from build123d import *

# Parameters (mm, degrees)
MAIN_BODY_DEPTH                        = 7
FLANG_CUT_RIGHT_DEPTH                  = 2.754419
FLANG_CUT_RIGHT_DIRECTION_2_REACH      = 15.268
FLANG_CUT_RIGHT_DIRECTION_2_END_RADIUS = 6
FLANG_CUT_LEFT_DEPTH                   = 2.754419
FLANG_CUT_LEFT_DIRECTION_2_REACH       = 17.116
FLANG_CUT_LEFT_DIRECTION_2_END_RADIUS  = 6
GUIDE_CUTS_DEPTH                       = 14.586908947


# Read off the part's stored shape, not the designer's step: CSK SLOT for M1.6 Countersunk Flat Head Screw9
with BuildPart() as part:
    # Sketch1 → main body (new body)
    with BuildSketch(Plane(origin=(0, 0, 0), x_dir=(1, 0, 0), z_dir=(0, 1, 0))):
        with BuildLine():
            Line((-0.042515674, 6.696868743), (-2.796934729, 6.696868743))
            ThreePointArc((-2.796934729, 6.696868743), (-1.044786012, 2.204228056), (3.447854676, 0.452079339))
            Line((3.447854676, 0.452079339), (3.447854676, 3.206498394))
            ThreePointArc((3.447854676, 3.206498394), (0.899757637, 4.148771704), (-0.042515674, 6.696868743))
        make_face()
        with BuildLine():
            Line((1.415300329, 6.696868743), (-0.042515674, 6.696868743))
            ThreePointArc((-0.042515674, 6.696868743), (0.899757637, 4.148771704), (3.447854676, 3.206498394))
            Line((3.447854676, 3.206498394), (3.447854676, 4.664314396))
            ThreePointArc((3.447854676, 4.664314396), (1.925062469, 5.174076537), (1.415300329, 6.696868743))
        make_face()
        with BuildLine():
            ThreePointArc((6.447854676, 6.446868743), (3.322947371, 9.694460438), (-0.042515674, 6.696868743))
            Line((-0.042515674, 6.696868743), (1.415300329, 6.696868743))
            ThreePointArc((1.415300329, 6.696868743), (1.907300469, 7.701647544), (2.897854676, 8.221692678))
            ThreePointArc((2.897854676, 8.221692678), (4.470646882, 7.719660949), (4.972678611, 6.146868743))
            ThreePointArc((4.972678611, 6.146868743), (4.452633477, 5.156314537), (3.447854676, 4.664314396))
            Line((3.447854676, 4.664314396), (3.447854676, 3.206498394))
            ThreePointArc((3.447854676, 3.206498394), (5.582702679, 4.238928527), (6.447854676, 6.446868743))
        make_face()
    extrude(amount=MAIN_BODY_DEPTH)

    # Sketch15 → flang cut right (cut)
    with BuildSketch(Plane(origin=(0, 0, -0.452079339), x_dir=(0, -1, 0), z_dir=(0, 0, 1))):
        Polygon((0, 3.447854676), (0, 2.712125029), (-7, 3.447854676), align=None)
    extrude(amount=-FLANG_CUT_RIGHT_DEPTH, mode=Mode.SUBTRACT)

    # flang cut right direction 2: up to this cylinder (the profile starts inside it)
    flang_cut_right_direction_2_end = Plane(origin=(3.197854676, 2.333333, -6.446868743), z_dir=(0, -1, 0)) * Cylinder(FLANG_CUT_RIGHT_DIRECTION_2_END_RADIUS, 43.536, mode=Mode.PRIVATE)
    # Sketch15 → flang cut right direction 2 (cut, up to the surface)
    with BuildSketch(Plane(origin=(0, 0, -0.452079339), x_dir=(0, -1, 0), z_dir=(0, 0, 1)), mode=Mode.PRIVATE) as flang_cut_right_direction_2_sk1:
        Polygon((0, 3.447854676), (0, 2.712125029), (-7, 3.447854676), align=None)
    flang_cut_right_direction_2_tool1 = extrude(flang_cut_right_direction_2_sk1.sketch, amount=FLANG_CUT_RIGHT_DIRECTION_2_REACH, mode=Mode.PRIVATE) & flang_cut_right_direction_2_end
    add(flang_cut_right_direction_2_tool1.solids().sort_by_distance((3.202611, 2.333333, -0.452079))[0], mode=Mode.SUBTRACT)

    # Sketch13 → flang cut left (cut)
    with BuildSketch(Plane(origin=(-2.796934729, 0, 0), x_dir=(0, 0, -1), z_dir=(1, 0, 0))):
        Polygon((6.696868743, 0), (6.696868743, 7), (5.7130829, 0), align=None)
    extrude(amount=FLANG_CUT_LEFT_DEPTH, mode=Mode.SUBTRACT)

    # flang cut left direction 2: up to this cylinder (the profile starts inside it)
    flang_cut_left_direction_2_end = Plane(origin=(3.197854676, 2.333333, -6.446868743), z_dir=(0, -1, 0)) * Cylinder(FLANG_CUT_LEFT_DIRECTION_2_END_RADIUS, 47.232, mode=Mode.PRIVATE)
    # Sketch13 → flang cut left direction 2 (cut, up to the surface)
    with BuildSketch(Plane(origin=(-2.796934729, 0, 0), x_dir=(0, 0, -1), z_dir=(1, 0, 0)), mode=Mode.PRIVATE) as flang_cut_left_direction_2_sk1:
        Polygon((6.696868743, 0), (6.696868743, 7), (5.7130829, 0), align=None)
    flang_cut_left_direction_2_tool1 = extrude(flang_cut_left_direction_2_sk1.sketch, amount=-FLANG_CUT_LEFT_DIRECTION_2_REACH, mode=Mode.PRIVATE) & flang_cut_left_direction_2_end
    add(flang_cut_left_direction_2_tool1.solids().sort_by_distance((-2.796935, 2.333333, -6.36894))[0], mode=Mode.SUBTRACT)

    # CSK SLOT for M1.6 Countersunk Flat H 2 → CSK SLOT for M1.6 Countersunk Flat Head Screw9 (revolve, cut)
    with BuildSketch(Plane(origin=(-1.673520994, 3.5, -1.59907768), x_dir=(0.723004631868789, 0, 0.6908431821305592), z_dir=(0, 1, 0))):
        Polygon((0.9, 4.170332063), (0.9, 5.425223714), (0, 5.425223714), (0, 0.870183673), (1.8, 0.870183673), (1.8, 3.270332063), align=None)
    revolve(axis=Axis((-1.673520994, 3.5, -1.59907768), (0.6908431821305593, 0, -0.7230046318687892)), mode=Mode.SUBTRACT)

    # Sketch11 → guide cuts (cut, through all)
    with BuildSketch(Plane.XZ):
        with BuildLine():
            Line((1.060664016, -5.013453966), (1.614472941, -5.59077162))
            ThreePointArc((1.614472941, -5.59077162), (1.951784592, -5.147904022), (2.408284716, -4.829284347))
            Line((2.408284716, -4.829284347), (1.85447579, -4.251966693))
            Line((1.85447579, -4.251966693), (1.060664016, -5.013453966))
        make_face()
        with BuildLine():
            Line((5.335045336, -7.88028352), (4.78123641, -7.302965866))
            ThreePointArc((4.78123641, -7.302965866), (4.443924759, -7.745833465), (3.987424635, -8.064453139))
            Line((3.987424635, -8.064453139), (4.541233561, -8.641770793))
            Line((4.541233561, -8.641770793), (5.335045336, -7.88028352))
        make_face()
    extrude(amount=-GUIDE_CUTS_DEPTH, mode=Mode.SUBTRACT)


solid = part.part
Could you check a few things on this model? Use its own coordinates, in mm. A direction names the side the tool comes from. Give positions to 0.01 mm unless a question says otherwise; leave off trailing zeros. Order: outer loops, then holes, each group sorted by start corner. A loop starts at its lowest first (then second) coordinate and runs counter-clockwise, first axis right, second up. Notation, with made-up numbers: (28, 43.5) - (35, 43.5) arc R13 ccw to (35, 49.5) - close; hole circle Ø10 at (48, -14). An arc over 180 degrees is marked (long way). One line per question, with ' | ' between items. Start each with the question number.
Item 1: I need wall thicknesses on probe 1 along Z at (x, y) = (4.5, 4.5); probe 2 along X at (y, z) = (2.5, -6.25); probe 3 along X at (y, z) = (2.75, -7). Which ranges of each line are inside material? Lowest first, please. Write a range as [from, to].
Item 2: Thinking about a two-plate mould opening in Y: for faces 3 (the flat face through (-1.4, 3.55, -6.21)), 4 (the cylindrical face through (1.01, 2.96, -1.92)), 5 (the flat face through (2, 7, -4)), 6 (the flat face through (-0.043, 2, -6.4)), which applies, pulls with the +Y half, pulls with the -Y half, needs draft (parallel to the pull), parting line crosses it, or undercut?
Item 3: I want a section at A-A on z = -7.75. Write out the boundary of the cut face in (x, y), then the cut area to 3 significant figures.
Item 4: I'm going to push flat-ended pins straight in: pin 1 Ø0.8 at (y, z) = (5, -6) entering from -X; pin 2 Ø1.5 at (y, z) = (1, -8) entering from +X; pin 3 Ø1.5 at (x, y) = (-1.5, 2) entering from +Z; pin 4 Ø2 at (x, y) = (5.5, 1.5) entering from -Z. Where does each tip first touch, or does it pass through?
Item 5: I want a section at D-D on y = 5.75. Write out the boundary of the cut face in (x, z), then the cut area to 3 significant figures.
Item 6: I want a section at B-B on x = 4.25. Write out the boundary of the cut face in (y, z), then the cut area to 3 significant figures.
Item 7: I want a section at C-C on y = 0.75. Write out the boundary of the cut face in (x, z).
Item 8: For faces 1 (the flat face through (0.8, 0, -5.1)), 2 (the flat face through (3.075, 3.451, -1.807)), which set-ups out of +Z, -Z, +X, -X, +Y, -Y let a thin tool reach every point of the face, with its end or its side?
Verdict:
1) probe 1: [-9.42, -8.6], [-5.2, -3.47] | probe 2: [-0.04, 1.41], [4.99, 6.44] | probe 3: [0, 1.48], [4.91, 6.4]
2) face 3: pulls with the -Y half | face 4: undercut | face 5: pulls with the +Y half | face 6: needs draft
3) outline: (0.22, 0) - (1.96, 0) - (1.96, 7) - (0.22, 7) - close; (5.21, 0) - (6.18, 0) - (6.18, 7) - (5.21, 7) - close | area: 18.9 mm^2
4) pin 1: x = -2.8 | pin 2: x = 6.35 | pin 3: z = -1.97 | pin 4: z = -9.42
5) outline: (-2.8, -6.52) - (-0.04, -6.52) - (-0.04, -6.7) arc R3.25 ccw (long way) to (3.45, -3.21) - (3.32, -3.21) - (3.32, -0.45) arc R6 ccw to start; hole (1.06, -5.01) - (1.61, -5.59) arc R1.8 ccw to (3.99, -8.06) - (4.54, -8.64) - (5.34, -7.88) - (4.78, -7.3) arc R1.8 ccw to (2.41, -4.83) - (1.85, -4.25) - close | area: 41.9 mm^2
6) outline: (0, -9.52) - (7, -9.52) - (7, -8.34) - (0, -8.34) - close; (0, -4.99) - (7, -4.99) - (7, -3.37) - (0, -3.37) - close | area: 19.6 mm^2
7) outline: (-2.77, -5.82) - (-0.04, -5.82) - (-0.04, -6.7) arc R3.25 ccw (long way) to (3.45, -3.21) - (2.79, -3.21) - (2.79, -0.46) arc R6 ccw to start; hole (1.06, -5.01) - (1.61, -5.59) arc R1.8 ccw to (3.99, -8.06) - (4.54, -8.64) - (5.34, -7.88) - (4.78, -7.3) arc R1.8 ccw to (2.41, -4.83) - (1.85, -4.25) - close
8) face 1: +Z, -Z, +X, -X, -Y | face 2: +Z, +X, -Y
